```python
from build123d import *

# Parameters (mm, degrees)
SKETCH2_R               = 15
BOSS_EXTRUDE2_DEPTH     = 140
SKETCH4_W               = 50
SKETCH4_H               = 50
BOSS_EXTRUDE3_DEPTH     = 89.61
FILLET1_R               = 5
FILLET3_R               = 10
SKETCH6_W               = 49.61
SKETCH6_H               = 30
CUT_EXTRUDE1_DEPTH      = 44.805
CUT_EXTRUDE5_DEPTH      = 193.878075737
CUT_EXTRUDE5_DEPTH_BACK = 193.878075737
SKETCH7_R               = 5


with BuildPart() as part:
    # Sketch2 → Boss-Extrude2 (new body)
    with BuildSketch(Plane.XY):
        Circle(SKETCH2_R)
    extrude(amount=BOSS_EXTRUDE2_DEPTH)

    # Sketch4 → Boss-Extrude3 (add)
    with BuildSketch(Plane.XY.offset(100)):
        Rectangle(SKETCH4_W, SKETCH4_H)
    extrude(amount=BOSS_EXTRUDE3_DEPTH)

    # Fillet1
    fillet1_edges = [part.edges().sort_by_distance(p)[0] for p in [
        (25, 0, 100),
        (0, 25, 100),
        (-25, 0, 100),
        (0, -25, 100),
    ]]
    fillet(fillet1_edges, radius=FILLET1_R)

    # Fillet3
    # the kernel refuses this fillet: 10 mm, written as the material it takes off along each edge
    with BuildSketch(Plane(origin=(15, 15, 100), x_dir=(0, 1, 0), z_dir=(-1, 0, 0))) as fillet3_piece_1:
        with BuildLine():
            CenterArc((5, -5), 5, 0, 90)
            Line((10, -5), (10, 0))
            Line((10, 0), (5, 0))
        make_face()
    revolve(axis=Axis((15, 15, 100), (0, 0, -1)), revolution_arc=90, mode=Mode.SUBTRACT)
    with BuildSketch(Plane(origin=(15, -15, 100), x_dir=(1, 0, 0), z_dir=(0, 1, 0))) as fillet3_piece_2:
        with BuildLine():
            CenterArc((5, -5), 5, 0, 90)
            Line((10, -5), (10, 0))
            Line((10, 0), (5, 0))
        make_face()
    revolve(axis=Axis((15, -15, 100), (0, 0, -1)), revolution_arc=90, mode=Mode.SUBTRACT)
    with BuildSketch(Plane(origin=(-15, 15, 100), x_dir=(-1, 0, 0), z_dir=(0, -1, 0))) as fillet3_piece_3:
        with BuildLine():
            CenterArc((5, -5), 5, 0, 90)
            Line((10, -5), (10, 0))
            Line((10, 0), (5, 0))
        make_face()
    revolve(axis=Axis((-15, 15, 100), (0, 0, -1)), revolution_arc=90, mode=Mode.SUBTRACT)
    with BuildSketch(Plane(origin=(-15, -15, 100), x_dir=(0, -1, 0), z_dir=(1, 0, 0))) as fillet3_piece_4:
        with BuildLine():
            CenterArc((5, -5), 5, 0, 90)
            Line((10, -5), (10, 0))
            Line((10, 0), (5, 0))
        make_face()
    revolve(axis=Axis((-15, -15, 100), (0, 0, -1)), revolution_arc=90, mode=Mode.SUBTRACT)
    with BuildSketch(Plane(origin=(25, -25, 100), x_dir=(0, 1, 0), z_dir=(0, 0, 1)), Plane(origin=(-25, -25, 100), x_dir=(1, 0, 0), z_dir=(0, 0, 1))) as fillet3_piece_5:
        with BuildLine():
            CenterArc((FILLET3_R, FILLET3_R), FILLET3_R, 180, 90)
            Line((0, FILLET3_R), (0, 0))
            Line((0, 0), (FILLET3_R, 0))
        make_face()
    extrude(amount=114.61, mode=Mode.SUBTRACT)
    with BuildSketch(Plane(origin=(25, 25, 100), x_dir=(0, -1, 0), z_dir=(0, 0, 1)), Plane(origin=(-25, 25, 100), x_dir=(1, 0, 0), z_dir=(0, 0, 1))) as fillet3_piece_6:
        with BuildLine():
            CenterArc((FILLET3_R, -FILLET3_R), FILLET3_R, 90, 90)
            Line((0, -FILLET3_R), (0, 0))
            Line((0, 0), (FILLET3_R, 0))
        make_face()
    extrude(amount=114.61, mode=Mode.SUBTRACT)

    # Sketch6 → Cut-Extrude1 (cut, symmetric)
    with BuildSketch(Plane(origin=(0, 0, 0), x_dir=(0, 0, -1), z_dir=(1, 0, 0))):
        with Locations((-164.805, 0)):
            Rectangle(SKETCH6_W, SKETCH6_H)
    extrude(amount=CUT_EXTRUDE1_DEPTH, both=True, mode=Mode.SUBTRACT)

    # Sketch7 → Cut-Extrude5 (cut, two sides: drawn at the far end of the back side and taken through both)
    with BuildSketch(Plane(origin=(0, 0, 0), x_dir=(1, 0, 0), z_dir=(0, 1, 0)).offset(-CUT_EXTRUDE5_DEPTH_BACK)):
        with Locations(Location((0, -175, 0), (0, 0, 270))):
            Circle(SKETCH7_R)
        with BuildLine():
            Line((-2.228917094, -189.61), (2.228917094, -189.61))
            ThreePointArc((2.228917094, -189.61), (4.246928068, -188.829826954), (5.21534053, -186.895087804))
            ThreePointArc((5.21534053, -186.895087804), (11.515192631, -161.931906551), (25, -140))
            ThreePointArc((25, -140), (0, -208.138826335), (-25, -140))
            ThreePointArc((-25, -140), (-11.515192631, -161.931906551), (-5.21534053, -186.895087804))
            ThreePointArc((-5.21534053, -186.895087804), (-4.246928068, -188.829826954), (-2.228917094, -189.61))
        make_face()
    extrude(amount=CUT_EXTRUDE5_DEPTH + CUT_EXTRUDE5_DEPTH_BACK, mode=Mode.SUBTRACT)


solid = part.part
```
Verification items for the finished model (mm, model axes). A direction names the side the tool comes from. Give positions to 0.01 mm unless a question says otherwise; leave off trailing zeros. Loops run counter-clockwise (first coordinate to the right, second up) from the corner with the lowest first, then second, coordinate; pieces in that order, holes last.
1. Section check A-A, the plane x = 0. Enter the section's corners in (y, z), then the cut area to 3 significant figures.
2. Mould release check, pull along Z, two halves, no side actions. Record for faces 1 (the cylindrical face through (23, 0, 101)), 2 (the flat face through (0, 0, 140)), 3 (the cylindrical face through (0, -20, 170)): released by +Z, released by -Z, zero draft, split by the parting line, or undercut.
3. Section check D-D, the plane z = 123.5. Enter the section's corners in (x, y).
4. Set-up check for faces 4 (the flat face through (9, 14, 100)), 5 (the flat face through (0, 20, 189.61)): record each of +Z, -Z, +X, -X, +Y, -Y from which the full face is reachable in a straight line by a thin tool's end or side.
5. Section check B-B, the plane z = 175. Enter the section's corners in (x, y).
6. Section check C-C, the plane y = 0. Enter the section's corners in (x, z).
7. Go/stop test with flat-tipped pins: pin 1 Ø1 at (x, y) = (19, 0.5) entering from -Z; pin 2 Ø2 at (y, z) = (16.5, 131) entering from +X; pin 3 Ø3 at (x, z) = (4, 76.5) entering from -Y; pin 4 Ø1.5 at (x, z) = (16.5, 38) entering from -Y. Record where each tip stops, or that it passes through.
8. Thickness scan on line 1 (Z direction, x = 0, y = -18); line 2 (Z direction, x = -11.5, y = -1); line 3 (Y direction, x = 0.5, z = 84). Record the ranges inside material, lowest first.
Geometry says:
1. outline: (-25, 105) arc R5 ccw to (-20, 100) - (-15, 100) - (-15, 0) - (15, 0) - (15, 100) - (20, 100) arc R5 ccw to (25, 105) - (25, 170) - (15, 170) - (15, 140) - (-15, 140) - (-15, 170) - (-25, 170) - close; (-25, 180) - (-15, 180) - (-15, 189.61) - (-25, 189.61) - close; (15, 180) - (25, 180) - (25, 189.61) - (15, 189.61) - close
1. area: 5,780 mm2
2. face 1: released by -Z
2. face 2: released by +Z
2. face 3: undercut
3. outline: (-25, -15) arc R10 ccw to (-15, -25) - (15, -25) arc R10 ccw to (25, -15) - (25, 15) arc R10 ccw to (15, 25) - (-15, 25) arc R10 ccw to (-25, 15) - close
4. face 4: -Z
4. face 5: +Z, +X, -X, +Y, -Y
5. outline: (-7.21, -25) - (-5, -25) - (-5, -15) - (-7.21, -15) - close; (-7.21, 15) - (-5, 15) - (-5, 25) - (-7.21, 25) - close; (5, -25) - (7.21, -25) - (7.21, -15) - (5, -15) - close; (5, 15) - (7.21, 15) - (7.21, 25) - (5, 25) - close
6. outline: (-25, 105) arc R5 ccw to (-20, 100) - (-15, 100) - (-15, 0) - (15, 0) - (15, 100) - (20, 100) arc R5 ccw to (25, 105) - (25, 140) - (-25, 140) - close
7. pin 1: stops at z = 100
7. pin 2: stops at x = 24.99
7. pin 3: stops at y = -14.79
7. pin 4: passes through
8. line 1: z = 100 to 170, 180 to 189.61
8. line 2: z = 0 to 140
8. line 3: y = -14.99 to 14.99
